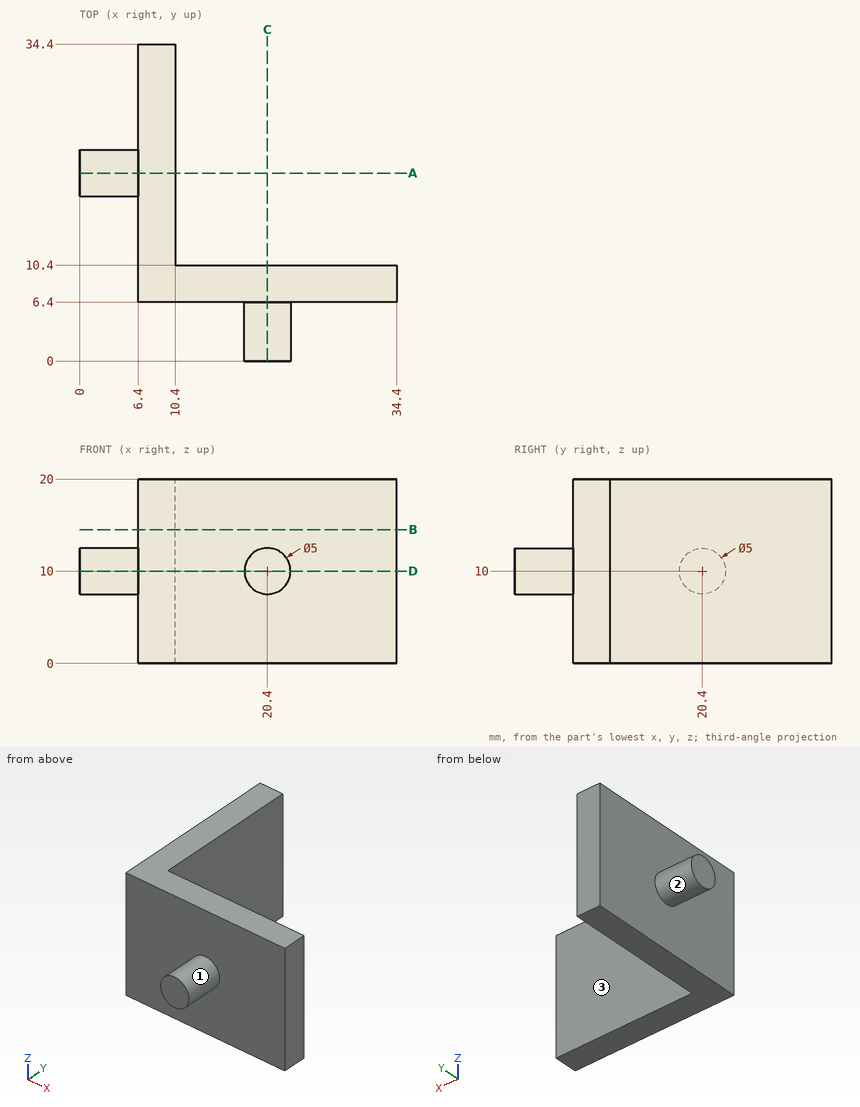
Answer from the drawing. Dimensions are ordinates in mm from the lowest x, y and z of the part. A direction names the side the tool comes from. Give positions to 0.01 mm unless a question says otherwise; leave off trailing zeros. Loops run counter-clockwise (first coordinate to the right, second up) from the corner with the lowest first, then second, coordinate; pieces in that order, holes last.
Item 1: For the marked faces 1, 2 and 3, determine the directions among +Z, -Z, +X, -X, +Y, -Y from which every point of the face is accessible in a straight line to the end or side of a thin tool.
Item 2: Each of these flat-tipped pins is pushed along its axis until it touches: pin 1 Ø4 at (y, z) = (15, 3.5) entering from -X; pin 2 Ø10 at (x, z) = (21, 14) entering from +Y; pin 3 Ø10 at (y, z) = (16, 5) entering from +X. Where does it stop, or does it pass through?
Item 3: The part is cut by section A-A (y = 20.4). Write down the section's boundary in (x, z), and give its area (3 significant figures).
Item 4: The part is cut by section B-B (z = 14.5). Write down the section's boundary in (x, y), and give its area (3 significant figures).
Item 5: The part is cut by section D-D (z = 10). Write down the section's boundary in (x, y).
Item 6: Find the intervals of material crossed by line 1 along X through (y, z) = (29, 1.5); line 2 along Y through (x, z) = (8, 17.25), in increasing order.
Taken from the geometry:
1. face 1: -Y
1. face 2: -X
1. face 3: +Z, -Z, +X, +Y
2. pin 1: stops at x = 6.4
2. pin 2: stops at y = 10.4
2. pin 3: stops at x = 10.4
3. outline: (0, 7.5) - (6.4, 7.5) - (6.4, 0) - (10.4, 0) - (10.4, 20) - (6.4, 20) - (6.4, 12.5) - (0, 12.5) - close
3. area: 112 mm2
4. outline: (6.4, 6.4) - (34.4, 6.4) - (34.4, 10.4) - (10.4, 10.4) - (10.4, 34.4) - (6.4, 34.4) - close
4. area: 208 mm2
5. outline: (0, 17.9) - (6.4, 17.9) - (6.4, 6.4) - (17.9, 6.4) - (17.9, 0) - (22.9, 0) - (22.9, 6.4) - (34.4, 6.4) - (34.4, 10.4) - (10.4, 10.4) - (10.4, 34.4) - (6.4, 34.4) - (6.4, 22.9) - (0, 22.9) - close
6. line 1: x = 6.4 to 10.4
6. line 2: y = 6.4 to 34.4
